Design review of the part built by this model. Coordinates are the model's own, in mm. Face numbers are marked on the shaded views. A direction names the side the tool comes from. Coordinates: 2 decimals unless noted, no trailing zeros. Write each loop counter-clockwise with the first axis right and the second up, starting at its lowest first coordinate (ties: lowest second). Pieces come first, ordered by that corner, then holes.
```python
from build123d import *

# Parameters (mm, degrees)
SKETCH1_R           = 24.9555
SKETCH1_R_2         = 23.368
BOSS_EXTRUDE1_DEPTH = 3.175
BOSS_EXTRUDE2_DEPTH = 3.175
FILLET1_R           = 1.6002


with BuildPart() as part:
    # Sketch1 → Boss-Extrude1 (new body)
    with BuildSketch(Plane.XY):
        Circle(SKETCH1_R)
        Circle(SKETCH1_R_2, mode=Mode.SUBTRACT)
    extrude(amount=BOSS_EXTRUDE1_DEPTH)

    # Sketch2 → Boss-Extrude2 (add, through all)
    with BuildSketch(Plane.XY.offset(3.175)):
        with BuildLine():
            Line((-14.063213461, 18.662514599), (-10.700271112, 14.199739369))
            Line((-10.700271112, 14.199739369), (-1.492452747, 14.199739369))
            Line((-1.492452747, 14.199739369), (-2.44262113, 23.239987651))
            ThreePointArc((-2.44262113, 23.239987651), (-8.564400666, 21.741997729), (-14.063213461, 18.662514599))
        make_face()
    extrude(amount=-BOSS_EXTRUDE2_DEPTH)

    # Fillet1
    fillet1_edges = [part.edges().sort_by_distance(p)[0] for p in [
        (-14.063213461, 18.662514599, 1.5875),
        (-2.44262113, 23.239987651, 1.5875),
        (-1.492452747, 14.199739369, 1.5875),
        (-10.700271112, 14.199739369, 1.5875),
    ]]
    fillet(fillet1_edges, radius=FILLET1_R)


solid = part.part
```
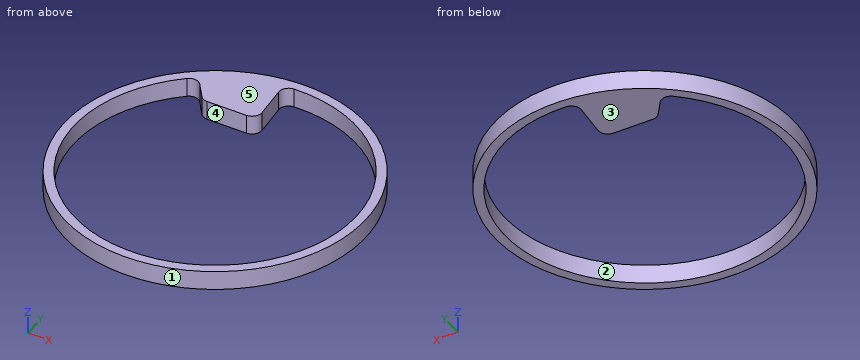
(1) Consider section A-A (x = 0). Give the boundary of the cut face in (y, z) (1 decimal).
(2) For the marked faces 4 and 5, list the 3-axis set-ups (+Z, -Z, +X, -X, +Y, -Y) from which the entire face can be reached by the end or side of a thin tool; tool diameter is ignored.
(3) Consider section C-C (z = 1.3). Give the boundary of the cut face in (x, y).
(4) Wall thickness on line 1 (Y direction, x = 0, z = 1.8); line 2 (X direction, y = 0.5, z = 1.7); line 3 (X direction, y = 6, z = 0.4): over which ranges is each line inside the solid? List them lowest first.
(5) Insertion check: pin 1 Ø1.5 at (y, z) = (4.5, 1.5) entering from -X; pin 2 Ø1.6 at (x, z) = (-6, 2) entering from -Y; pin 3 Ø12 at (x, y) = (3, 10) entering from -Z (3 decimals). Each pin has a flat end and moves straight along its axis. Give the tip position at first contact, or say it passes through.
(6) Mouldability with a two-part tool opening along Y and no side actions: class the marked faces 1, 2 and 3 as +Y half, -Y half, draft (parallel to the pull), parting line (faces both ways), or undercut.
Results:
1. outline: (-25, 0) - (-23.4, 0) - (-23.4, 3.2) - (-25, 3.2) - close; (23.4, 0) - (25, 0) - (25, 3.2) - (23.4, 3.2) - close
2. face 4: +Z, -Z
2. face 5: +Z, +X, -X, +Y, -Y
3. outline: circle Ø49.91 at (0, 0); hole (-15.4, 17.58) arc R23.37 ccw (long way) to (-0.73, 23.36) arc R1.6 ccw to (-2.27, 21.59) - (-1.68, 15.97) arc R1.6 cw to (-3.27, 14.2) - (-9.9, 14.2) arc R1.6 cw to (-11.18, 14.84) - (-13.06, 17.34) arc R1.6 ccw to start
4. line 1: y = -24.96 to -23.37, 23.37 to 24.96
4. line 2: x = -24.95 to -23.36, 23.36 to 24.95
4. line 3: x = -24.22 to -22.58, 22.58 to 24.22
5. pin 1: stops at x = -24.67
5. pin 2: stops at y = -24.41
5. pin 3: passes through
6. face 1: parting line
6. face 2: undercut
6. face 3: draft
